Could you check a few things on this model? Use its own coordinates, in mm. Face numbers are marked on the shaded views. A direction names the side the tool comes from. Round coordinates to 2 decimals unless told otherwise and drop trailing zeros. Loops run counter-clockwise (first coordinate to the right, second up) from the corner with the lowest first, then second, coordinate; pieces in that order, holes last.
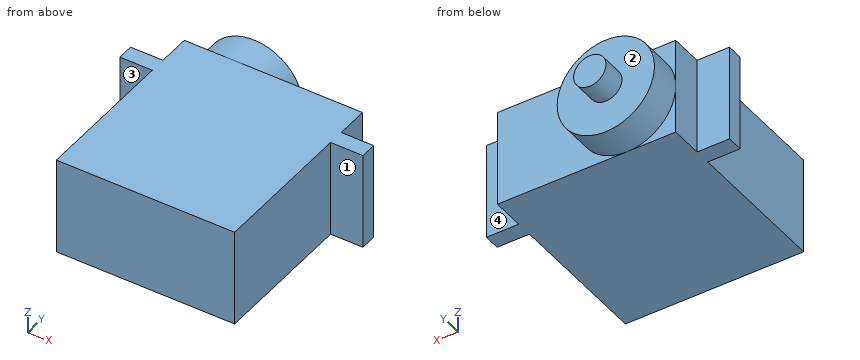
from build123d import *

# Parameters (mm, degrees)
SKETCH1_W           = 22
SKETCH1_H           = 24
BOSS_EXTRUDE1_DEPTH = 12
BOSS_EXTRUDE2_START = 4
SKETCH2_W           = 12
SKETCH2_H           = 2
BOSS_EXTRUDE2_DEPTH = 30
SKETCH3_R           = 6
BOSS_EXTRUDE3_DEPTH = 4
SKETCH4_R           = 2
BOSS_EXTRUDE4_DEPTH = 3


with BuildPart() as part:
    # Sketch1 → Boss-Extrude1 (new body)
    with BuildSketch(Plane.XY):
        Rectangle(SKETCH1_W, SKETCH1_H)
    extrude(amount=BOSS_EXTRUDE1_DEPTH)

    # Sketch2 → Boss-Extrude2 (add)
    with BuildSketch(Plane.ZY.offset(11).offset(BOSS_EXTRUDE2_START)):
        with Locations((6, 7)):
            Rectangle(SKETCH2_W, SKETCH2_H)
    extrude(amount=-BOSS_EXTRUDE2_DEPTH)

    # Sketch3 → Boss-Extrude3 (add)
    with BuildSketch(Plane(origin=(0, 12, 0), x_dir=(1, 0, 0), z_dir=(0, 1, 0))):
        with Locations((-5, -6)):
            Circle(SKETCH3_R)
    extrude(amount=BOSS_EXTRUDE3_DEPTH)

    # Sketch4 → Boss-Extrude4 (add)
    with BuildSketch(Plane(origin=(0, 16, 0), x_dir=(1, 0, 0), z_dir=(0, 1, 0))):
        with Locations((-5, -6)):
            Circle(SKETCH4_R)
    extrude(amount=BOSS_EXTRUDE4_DEPTH)


solid = part.part
Item 1: Will these pins go through, and if not, where does the flat tip stop? pin 1 (6 mm diameter, centred on y = -5.5, z = 5.5, fed in from -X); pin 2 (1.2 mm diameter, centred on x = -12.5, z = 7.5, fed in from -Y); pin 3 (1.8 mm diameter, centred on x = -9, z = 3.5, fed in from +Y).
Results list:
pin 1: stops at x = -11
pin 2: stops at y = 6
pin 3: stops at y = 16
Item 2: If I drill on line 1 along Y through (x, z) = (-12.25, 10.25); line 2 along X through (y, z) = (-7, 3.5); line 3 along Y through (x, z) = (-10, 8.5), over which ranges is the centre line in solid material (lowest first)?
Results list:
line 1: y = 6 to 8
line 2: x = -11 to 11
line 3: y = -12 to 16
Item 3: If we section it at D-D, the plane z = 7.25: Please give me the cut outline in (x, y).
Results list:
outline: (-15, 6) - (-11, 6) - (-11, -12) - (11, -12) - (11, 6) - (15, 6) - (15, 8) - (11, 8) - (11, 12) - (0.87, 12) - (0.87, 16) - (-3.44, 16) - (-3.44, 19) - (-6.56, 19) - (-6.56, 16) - (-10.87, 16) - (-10.87, 12) - (-11, 12) - (-11, 8) - (-15, 8) - close
Item 4: If we section it at C-C, the plane x = 9: Please give me the cut outline in (y, z), then the cut area to 3 significant figures.
Results list:
outline: (-12, 0) - (12, 0) - (12, 12) - (-12, 12) - close
area: 288 mm2
Item 5: If we section it at A-A, the plane z = 3.25: Please give me the cut outline in (x, y).
Results list:
outline: (-15, 6) - (-11, 6) - (-11, -12) - (11, -12) - (11, 6) - (15, 6) - (15, 8) - (11, 8) - (11, 12) - (0.33, 12) - (0.33, 16) - (-10.33, 16) - (-10.33, 12) - (-11, 12) - (-11, 8) - (-15, 8) - close
Item 6: If we section it at B-B, the plane y = 10.5: Please give me the cut outline in (x, z).
Results list:
outline: (-11, 0) - (11, 0) - (11, 12) - (-11, 12) - close
Item 7: For the marked faces 1, 2, 3 and 4, which set-ups out of +Z, -Z, +X, -X, +Y, -Y let a thin tool reach every point of the face, with its end or its side?
Results list:
face 1: +Z, -Z, +X, -Y
face 2: +Y
face 3: +Z, -Z, -X, -Y
face 4: +Z, -Z, +X, +Y
